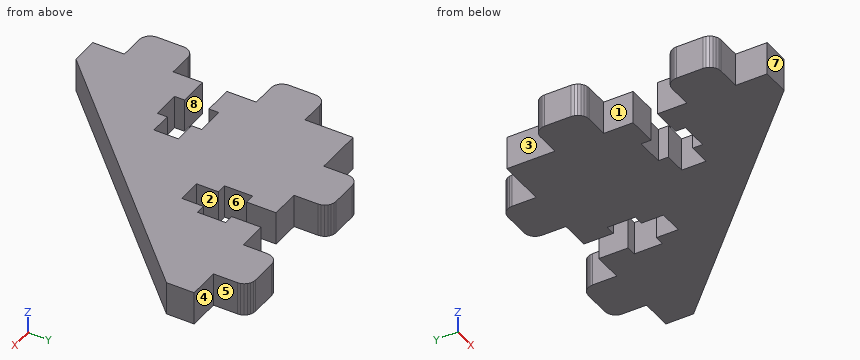
from build123d import *

# Parameters (mm, degrees)
RESSALTO_EXTRUS_O1_DEPTH = 6


with BuildPart() as part:
    # Model → Ressalto-extrusão1 (new body)
    with BuildSketch(Plane.XY):
        Polygon((37.969283539, 43.996209277), (41.919283362, 43.996209277), (41.919283362, 39.596204606), (37.969283539, 39.596204606), (37.969283539, 37.796206374), (32.869285775, 37.796206374), (32.869285775, 39.596204606), (27.569286953, 39.596204606), (27.569286953, 34.296207351), (23.219289062, 34.296207351), (22.701650972, 34.228059003), (22.219289062, 34.028258158), (21.8050755, 33.710420913), (21.487238254, 33.296207351), (21.287437409, 32.813845441), (21.219289062, 32.296207351), (21.219289062, 27.496212909), (21.287437409, 26.978574818), (21.487238254, 26.496212909), (21.8050755, 26.081999346), (22.219289062, 25.764162101), (22.701650972, 25.564361256), (23.219289062, 25.496212909), (27.569286953, 25.496212909), (27.569286953, 19.803247953), (32.573283526, 19.803247953), (74.566390822, 61.794924044), (74.566390822, 66.796199314), (68.869269338, 66.796199314), (68.869269338, 71.146197205), (68.80112099, 71.663835295), (68.601320145, 72.146197205), (68.2834829, 72.560410768), (67.869269338, 72.878248013), (67.386907428, 73.078048858), (66.869269338, 73.146197205), (62.069273373, 73.146197205), (61.551635282, 73.078048858), (61.069273373, 72.878248013), (60.65505981, 72.560410768), (60.337222565, 72.146197205), (60.13742172, 71.663835295), (60.069273373, 71.146197205), (60.069273373, 66.796199314), (54.769281366, 66.796199314), (54.769281366, 61.496200492), (56.569279598, 61.496200492), (56.569279598, 56.396202728), (54.769281366, 56.396202728), (54.769281366, 52.446202905), (50.369276694, 52.446202905), (50.369276694, 56.396202728), (48.569278462, 56.396202728), (48.569278462, 61.496200492), (50.369276694, 61.496200492), (50.369276694, 66.796199314), (45.069279439, 66.796199314), (45.069279439, 71.146197205), (45.001131092, 71.663835295), (44.801330247, 72.146197205), (44.483493001, 72.560410768), (44.069279439, 72.878248013), (43.586917529, 73.078048858), (43.069279439, 73.146197205), (38.269284997, 73.146197205), (37.751646907, 73.078048858), (37.269284997, 72.878248013), (36.855071435, 72.560410768), (36.537234189, 72.146197205), (36.337433344, 71.663835295), (36.269284997, 71.146197205), (36.269284997, 66.796199314), (27.569286953, 66.796199314), (27.569286953, 58.096197249), (23.219289062, 58.096197249), (22.701650972, 58.028048902), (22.219289062, 57.828248057), (21.8050755, 57.510410812), (21.487238254, 57.096197249), (21.287437409, 56.613835339), (21.219289062, 56.096197249), (21.219289062, 51.296201284), (21.287437409, 50.778563194), (21.487238254, 50.296201284), (21.8050755, 49.881987722), (22.219289062, 49.564150477), (22.701650972, 49.364349632), (23.219289062, 49.296201284), (27.569286953, 49.296201284), (27.569286953, 43.996209277), (32.869285775, 43.996209277), (32.869285775, 45.796207509), (37.969283539, 45.796207509), align=None)
    extrude(amount=RESSALTO_EXTRUS_O1_DEPTH)


solid = part.part
Could you check a few things on this model? Use its own coordinates, in mm. Face numbers are marked on the shaded views. A direction names the side the tool comes from. Round coordinates to 2 decimals unless told otherwise and drop trailing zeros. Write each loop counter-clockwise with the first axis right and the second up, starting at its lowest first coordinate (ties: lowest second). Pieces come first, ordered by that corner, then holes. Notation, with made-up numbers: (-22, 35) - (-16, 35) arc R20 ccw to (-16, 74) - close; hole circle Ø9 at (25.5, 75.25). An arc over 180 degrees is marked (long way). Put each result on its own line as item: value. Start each with the question number.
(1) Will these pins go through, and if not, where does the flat tip stop? pin 1 (0.5 mm diameter, centred on y = 45, z = 3.5, fed in from -X); pin 2 (1.5 mm diameter, centred on y = 33.5, z = 2, fed in from -X); pin 3 (2 mm diameter, centred on y = 69, z = 4, fed in from +X); pin 4 (5 mm diameter, centred on x = 34, y = 55, fed in from -Z).
(2) I want a section at B-B, the plane y = 65. Please give me the cut outline in (x, z).
(3) I want a section at D-D, the plane y = 36.5. Please give me the cut outline in (x, z).
(4) I want a section at A-A, the plane x = 30. Please give me the cut outline in (y, z), plus the area to 3 significant figures.
(5) I need wall thicknesses on probe 1 along X at (y, z) = (64, 3.15); probe 2 along X at (y, z) = (70.5, 4.75); probe 3 along Y at (x, z) = (32, 2). Which ranges of each line are inside material? Lowest first, please.
(6) I want a section at C-C, the plane x = 63. Please give me the cut outline in (y, z).
(7) Thinking about a two-plate mould opening in Y: for the marked faces 5, 6, 7 and 8, which applies, released by +Y, released by -Y, zero draft, split by the parting line, or undercut?
(8) For the marked faces 1, 2, 3 and 4, which set-ups out of +Z, -Z, +X, -X, +Y, -Y let a thin tool reach every point of the face, with its end or its side?
Here are the results:
1. pin 1: stops at x = 27.57
1. pin 2: stops at x = 21.28
1. pin 3: stops at x = 68.87
1. pin 4: stops at z = 0
2. outline: (27.57, 0) - (50.37, 0) - (50.37, 6) - (27.57, 6) - close; (54.77, 0) - (74.57, 0) - (74.57, 6) - (54.77, 6) - close
3. outline: (27.57, 0) - (49.27, 0) - (49.27, 6) - (27.57, 6) - close
4. outline: (19.8, 0) - (39.6, 0) - (39.6, 6) - (19.8, 6) - close; (44, 0) - (66.8, 0) - (66.8, 6) - (44, 6) - close
4. area: 256 mm^2
5. probe 1: x = 27.57 to 50.37, 54.77 to 74.57
5. probe 2: x = 36.27 to 45.07, 60.07 to 68.87
5. probe 3: y = 19.8 to 39.6, 44 to 66.8
6. outline: (50.23, 0) - (73.15, 0) - (73.15, 6) - (50.23, 6) - close
7. face 5: zero draft
7. face 6: undercut
7. face 7: released by -Y
7. face 8: undercut
8. face 1: +Z, -Z, -X
8. face 2: +Z, -Z, +Y
8. face 3: +Z, -Z, -X, +Y
8. face 4: +Z, -Z, +X, +Y
